from build123d import *

# Parameters (mm, degrees)
F0_R          = 15
F1_DEPTH      = 1
F1_DEPTH_BACK = 1
F2_R          = 1
F3_DEPTH      = 2
F3_DEPTH_BACK = 2
F3_TAPER_BACK = -30
F4_R          = 9
F4_R_2        = 7.5
F5_DEPTH      = 3
F6_DEPTH      = 5
F7_R          = 0.99999


# Not quite as in the source:
# - a fillet or chamfer is up to 0.001 mm smaller than in the source, because OpenCascade refuses the exact size


with BuildPart() as f1:
    # F0 (on Top) → F1 (new body, two sides)
    with BuildSketch(Plane.XY) as f1_sk:
        Circle(F0_R)
    extrude(amount=F1_DEPTH)
    extrude(f1_sk.sketch, amount=-F1_DEPTH_BACK)

    # F2 (on Top) → F3 (cut, two sides)
    with BuildSketch(Plane.XY) as f3_sk:
        with Locations((12, 0)):
            Circle(F2_R)
        with Locations((0, 12)):
            Circle(F2_R)
        with Locations((-12, 0)):
            Circle(F2_R)
        with Locations((0, -12)):
            Circle(F2_R)
    extrude(amount=-F3_DEPTH, mode=Mode.SUBTRACT)
    extrude(f3_sk.sketch, amount=F3_DEPTH_BACK, taper=F3_TAPER_BACK, mode=Mode.SUBTRACT)

    # F4 (on face) → F5 (join)
    with BuildSketch(Plane.XY.offset(1)):
        Circle(F4_R)
        Circle(F4_R_2, mode=Mode.SUBTRACT)
    extrude(amount=F5_DEPTH)

    # F6 (cut): a face of the model
    f6_faces = [f1.faces().sort_by_distance(p)[0] for p in [
        (0, 0, 1),
    ]]
    extrude(f6_faces, amount=-F6_DEPTH, mode=Mode.SUBTRACT)

    # F7 (radius 1 in the source; OpenCascade refuses exactly that, so slightly less here)
    f7_edges = [f1.edges().sort_by_distance(p)[0] for p in [
        (-15, 0, 1),
        (-9, 0, 1),
    ]]
    fillet(f7_edges, radius=F7_R)


solid = f1.part
Could you check a few things on this model? Use its own coordinates, in mm. A direction names the side the tool comes from. Round coordinates to 2 decimals unless told otherwise and drop trailing zeros. Loops run counter-clockwise (first coordinate to the right, second up) from the corner with the lowest first, then second, coordinate; pieces in that order, holes last. Notation, with made-up numbers: (2.5, 86) -> (16.5, 86) arc R30 ccw to (16.5, 123) -> close; hole circle Ø2 at (47, 89). An arc over 180 degrees is marked (long way). Use CSV: the item, a comma, the result in double quotes.
(1) Will these pins go through, and if not, where does the flat tip stop? pin 1 Ø2 at (x, y) = (-8, 11.5) entering from +Z; pin 2 Ø9 at (x, y) = (0, 0) entering from -Z; pin 3 Ø1.5 at (x, z) = (0, 1.5) entering from +Y; pin 4 Ø1.5 at (x, z) = (-8.5, 2.5) entering from -Y.
Return value:
pin 1,"stops at z = 1"
pin 2,"passes through"
pin 3,"stops at y = 14.66"
pin 4,"stops at y = -4.58"
(2) Suppose I cut it at C-C on z = 3. Write out the boundary of the cut face in (x, y).
Return value:
outline,"circle Ø18 at (0, 0); hole circle Ø15 at (0, 0)"
(3) If I drill on probe 1 along Y at (x, z) = (-12, 0); probe 2 along Z at (x, y) = (3, 13.5); probe 3 along Y at (x, z) = (3, 2.7), over which ranges is the centre line in solid material (lowest first)? Write a range as [from, to].
Return value:
probe 1,"y = [-9, -1], [1, 9]"
probe 2,"z = [-1, 1]"
probe 3,"y = [-8.49, -6.87], [6.87, 8.49]"
(4) For faces 4 (the cylindrical face through (11, 0, -0.5)), 5 (the cylindrical face through (-1.172, 8.923, 2.986)), which set-ups out of +Z, -Z, +X, -X, +Y, -Y let a thin tool reach every point of the face, with its end or its side?
Return value:
face 4,"+Z, -Z"
face 5,"+Z"
(5) Suppose I cut it at A-A on x = 0. Write out the boundary of the cut face in (y, z), plus the area to 3 significant figures.
Return value:
outline,"(-15, -1) -> (-13, -1) -> (-13, 0) -> (-13.58, 1) -> (-14, 1) arc R1 ccw to (-15, 0) -> close; (-11, -1) -> (-7.5, -1) -> (-7.5, 4) -> (-9, 4) -> (-9, 2) arc R1 cw to (-10, 1) -> (-10.42, 1) -> (-11, 0) -> close; (7.5, -1) -> (11, -1) -> (11, 0) -> (10.42, 1) -> (10, 1) arc R1 cw to (9, 2) -> (9, 4) -> (7.5, 4) -> close; (13, -1) -> (15, -1) -> (15, 0) arc R1 ccw to (14, 1) -> (13.58, 1) -> (13, 0) -> close"
area,"29.8 mm²"
(6) If we mould it in two halves opening along X, with no side actions, what happens to faces 1 (the cylindrical face through (-14.985, 0.66, -0.493)), 2 (the flat face through (9.3, -4.1, 1)), 3 (the cylindrical face through (-0.13, -11.01, -0.49))? For each: +X half, -X half, draft (parallel to the pull), parting line (faces both ways), or undercut.
Return value:
face 1,"parting line"
face 2,"draft"
face 3,"undercut"
(7) Suppose I cut it at B-B on y = 0. Give the number of separate pieces and of enclosed holes in the cut face, plus the area to 3 significant figures.
Return value:
separate pieces,"4"
enclosed holes,"0"
area,"29.8 mm²"
